Autodesk Inventor part; units mm, degrees
ref_plane "YZ Plane" through (0, 0, 0) normal (1, 0, 0) x (0, 1, 0)
ref_plane "XZ Plane" through (0, 0, 0) normal (0, 1, 0) x (-1, 0, 0)
ref_plane "XY Plane" through (0, 0, 0) normal (0, 0, 1) x (1, 0, 0)
sketch "Sketch1" plane through (0, 0, 0) normal (0, 0, 1) x (1, 0, 0)
  line L0 (0, 0) -> (80, 0)
  line L1 (80, 0) -> (80, 86)
  line L2 (80, 86) -> (0, 86)
  line L3 (0, 86) -> (0, 0)
  dimension "d0" = 80
  dimension "d1" = 86
extrude "Extrusion1" add sketch "Sketch1" along normal blind 15
sketch "Sketch2" plane through (0, 0, 15) normal (0, 0, 1) x (1, 0, 0)
  line L0 (0, 0) -> (0, 86)
  line L1 (80, 0) -> (0, 0)
  line L2 (80, 86) -> (80, 0)
  line L3 (0, 86) -> (80, 86)
  line L4 (0, 86) -> (10, 86)
  line L5 (10, 86) -> (10, 60)
  line L6 (10, 60) -> (0, 60)
  line L7 (0, 60) -> (0, 86)
  line L8 (70, 86) -> (80, 86)
  line L9 (80, 86) -> (80, 40)
  line L10 (80, 40) -> (70, 40)
  line L11 (70, 40) -> (70, 86)
  line L12 (54, 0) -> (80, 0)
  line L13 (80, 0) -> (80, 20)
  line L14 (80, 20) -> (54, 20)
  line L15 (54, 20) -> (54, 0)
  line L16 (0, 20) -> (26, 20)
  line L17 (26, 20) -> (26, 0)
  line L18 (26, 0) -> (0, 0)
  line L19 (0, 0) -> (0, 20)
  dimension "d4" = 20
  dimension "d5" = 20
  dimension "d6" = 20
  dimension "d7" = 10
  dimension "d8" = 10
  dimension "d9" = 40
  dimension "d10" = 28
  dimension "d11" = 26
extrude "Extrusion2" cut sketch "Sketch2" against normal blind 15 contours L0 L16 L17 L1 | L0 L3 L5 L6 | L15 L14 L2 L1 | L3 L2 L10 L11
sketch "Sketch3" plane through (0, 0, 15) normal (0, 0, 1) x (1, 0, 0)
  line L0 (10, 86) -> (10, 60)
  line L1 (10, 60) -> (0, 60)
  line L2 (0, 20) -> (0, 60)
  line L3 (0, 20) -> (26, 20)
  line L4 (26, 20) -> (26, 0)
  line L5 (54, 0) -> (26, 0)
  line L6 (54, 0) -> (54, 20)
  line L7 (54, 20) -> (80, 20)
  line L8 (80, 40) -> (80, 20)
  line L9 (80, 40) -> (70, 40)
  line L10 (70, 40) -> (70, 86)
  line L11 (10, 86) -> (70, 86)
  line L12 (0, 20) -> (10, 20)
  line L13 (10, 20) -> (10, 40)
  line L14 (10, 40) -> (0, 40)
  line L15 (0, 40) -> (0, 20)
  point P0 (0, 0)
  dimension "d14" = 10
  dimension "d15" = 20
extrude "Extrusion3" cut sketch "Sketch3" against normal blind 15 contours L14 L13 L3 L2
sketch "Sketch4" plane through (0, 0, 15) normal (0, 0, 1) x (1, 0, 0)
  line L0 (26, 20) -> (26, 0)
  line L1 (54, 0) -> (26, 0)
  line L2 (10, 86) -> (70, 86)
  line L3 (0, 40) -> (0, 60)
  point P0 (0, 0)
  point P1 (40, 72)
  point P2 (40, 14)
  dimension "d18" = 14
  dimension "d19" = 40
  dimension "d20" = 14
  dimension "d21" = 14
hole "Hole1" at (40, 72, 15) at (40, 14, 15) direction (0, 0, -1) diameter 14 depth 15 tip angle 118
sketch "Sketch5" plane through (0, 0, 15) normal (0, 0, 1) x (1, 0, 0)
  circle A0 centre (40, 72) radius 7
  line L0 (0, 40) -> (0, 60)
  point P0 (0, 0)
  point P1 (40, 43)
  dimension "d29" = 29
  dimension "d30" = 40
hole "Hole2" at (40, 43, 15) direction (0, 0, -1) diameter 14 depth 18 tip angle 118 counterbore diameter 22 counterbore depth 3
fillet "Fillet1" radius 14 2 edges at (26, 0, 7.5) (54, 0, 7.5)
sketch "Sketch6" plane through (0, 0, 15) normal (0, 0, 1) x (1, 0, 0)
  line L0 (70, 40) -> (80, 40)
  line L1 (80, 40) -> (80, 20)
  line L2 (80, 20) -> (70, 20)
  line L3 (70, 20) -> (70, 40)
  point P0 (0, 0)
extrude "Extrusion4" cut sketch "Sketch6" against normal blind 15
sketch "Sketch7" plane through (0, 60, 15) normal (0, 1, 0) x (1, 0, 0)
  line L0 (0, 15) -> (10, 15)
  line L1 (10, 0) -> (10, 15)
  point P0 (5, 7.5)
  dimension "d41" = 7.5
  dimension "d42" = 5
hole "Hole3" at (5, 60, 7.5) direction (0, -1, 0) diameter 6.647 depth 20 tip angle 118
chamfer "Chamfer1" distance 0.5 angle 45 2 edges at (5, 60, 4.1765) (5, 40, 4.1765)
sketch "Sketch8" plane through (0, 0, 15) normal (0, 0, 1) x (1, 0, 0)
  circle A0 centre (40, 72) radius 7
  line L0 (10, 86) -> (70, 86)
  point P0 (0, 0)
  point P1 (21, 76)
  point P2 (59, 76)
  dimension "d53" = 38
  dimension "d54" = 19
  dimension "d55" = 10
hole "Hole4" at (21, 76, 15) at (59, 76, 15) direction (0, 0, -1) diameter 4.917 depth 12 tip angle 118
chamfer "Chamfer2" distance 0.5 angle 45 2 edges at (21, 78.4585, 15) (59, 78.4585, 15)
sketch "Sketch9" plane through (70, 20, 15) normal (1, 0, 0) x (0, 0, -1)
  line L0 (15, 66) -> (15, 0)
  line L1 (0, 66) -> (15, 66)
  point P0 (15, -20)
  point P1 (7.5, 10)
  dimension "d66" = 7.5
  dimension "d67" = 56
hole "Hole5" at (70, 30, 7.5) direction (-1, 0, 0) diameter 4.917 depth 15 tip angle 118
chamfer "Chamfer3" distance 0.5 angle 45 1 edges at (70, 30, 9.9585)
sketch "Sketch10" plane through (10, 20, 15) normal (-1, 0, 0) x (0, 0, 1)
  line L0 (-15, 0) -> (-15, 20)
  line L1 (0, 0) -> (-15, 0)
  point P0 (-15, -20)
  point P1 (-7.5, 10)
  dimension "d78" = 10
  dimension "d79" = 7.5
hole "Hole6" at (10, 30, 7.5) direction (1, 0, 0) diameter 4.917 depth 15 tip angle 118
chamfer "Chamfer4" distance 0.5 angle 45 1 edges at (10, 30, 5.0415)
properties part number "PLACA COM FUROS COORDENADOS(13)" material "Carbon Steel"
Input: part model. Units: mm. Frame: model coordinates. A direction names the side the tool comes from. Coordinates: 2 decimals unless noted, no trailing zeros. Order: outer loops, then holes, each group sorted by start corner. A loop starts at its lowest first (then second) coordinate and runs counter-clockwise, first axis right, second up. Notation, with made-up numbers: M -16.75,68.25 L 42.25,68.25 A13 cw 42.25,78.25 Z; hole C 45,34 d11. An arc over 180 degrees is marked long. Answer in a Markdown table with one row per item.
(1) Section query A-A, the plane y = 72. Output: boundary loops of the cut face in (x, z).
Numbers:
| item | result |
|---|---|
| outline | M 10,0 L 33,0 L 33,15 L 10,15 Z; M 47,0 L 70,0 L 70,15 L 47,15 Z |
(2) Contact query for flat-ended pins moving along their axis: pin 1 Ø1 at (x, z) = (16.5, 13.5) entering from -Y; pin 2 Ø3 at (y, z) = (30, 7.5) entering from +X; pin 3 Ø16 at (x, y) = (40, 43) entering from +Z; pin 4 Ø11 at (x, y) = (40, 72) entering from -Z. Output: stop coordinate, or through.
Numbers:
| item | result |
|---|---|
| pin 1 | stops at y = 20 |
| pin 2 | stops at x = 54.42 |
| pin 3 | stops at z = 12 |
| pin 4 | passes through |
(3) Access query for faces 4 (the cylindrical face through (62.15, 32.4, 8.03)), 5 (the cylindrical face through (36.696, 32.508, 13.479)), 6 (the flat face through (54, 17, 8)), 7 (the cylindrical face through (17.85, 32.4, 6.97)), 8 (the flat face through (10, 30, 11)). Directions: +Z, -Z, +X, -X, +Y, -Y. A direction counts if a zero-diameter tool reaches every point of the face in a straight line with its end or side. Return the directions, or none.
Numbers:
| item | result |
|---|---|
| face 4 | +X |
| face 5 | +Z |
| face 6 | +Z, -Z, +X, -Y |
| face 7 | -X |
| face 8 | +Z, -Z, -X, -Y |
(4) Section query C-C, the plane x = 17. Output: boundary loops of the cut face in (y, z), plus the area to 3 significant figures.
Numbers:
| item | result |
|---|---|
| outline | M 20,0 L 86,0 L 86,15 L 20,15 Z; hole C 30,7.5 d4.92 |
| area | 971 mm^2 |
(5) Section query B-B, the plane x = 42.5. Output: boundary loops of the cut face in (y, z) (3 decimals), plus the area to 3 significant figures.
Numbers:
| item | result |
|---|---|
| outline | M 0.225,0 L 7.462,0 L 7.462,15 L 0.225,15 Z; M 20.538,0 L 36.462,0 L 36.462,12 L 32.288,12 L 32.288,15 L 20.538,15 Z; M 49.538,0 L 65.462,0 L 65.462,15 L 53.712,15 L 53.712,12 L 49.538,12 Z; M 78.538,0 L 86,0 L 86,15 L 78.538,15 Z |
| area | 673 mm^2 |
(6) Draft query along Y for faces 1 (the cylindrical face through (35.27, 77.16, 7.4)), 2 (the cylindrical face through (30.2, 4, 7.4)), 3 (the flat face through (35, 53, 0)). Return one class per face: pulls with the +Y half, pulls with the -Y half, needs draft (parallel to the pull), parting line crosses it, or undercut.
Numbers:
| item | result |
|---|---|
| face 1 | undercut |
| face 2 | pulls with the -Y half |
| face 3 | needs draft |
(7) Section query D-D, the plane y = 53. Output: boundary loops of the cut face in (x, z), plus the area to 3 significant figures.
Numbers:
| item | result |
|---|---|
| outline | M 0,0 L 70,0 L 70,15 L 44.58,15 L 44.58,12 L 35.42,12 L 35.42,15 L 0,15 Z; hole C 5,7.5 d6.65 |
| area | 988 mm^2 |
(8) Material intervals for line 1 (Y direction, x = 40, z = 4.5); line 2 (X direction, y = 72, z = 8.5); line 3 (X direction, y = 77.5, z = 14.25), sorted ascending. Write a range as [from, to].
Numbers:
| item | result |
|---|---|
| line 1 | y = [0, 7], [21, 36], [50, 65], [79, 86] |
| line 2 | x = [10, 33], [47, 70] |
| line 3 | x = [10, 19.05], [22.95, 35.67], [44.33, 57.05], [60.95, 70] |
